Build history of the part. All positions in model axes, mm. A direction names the side the tool comes from. Give positions to 0.01 mm unless a question says otherwise; leave off trailing zeros. Order: outer loops, then holes, each group sorted by start corner. A loop starts at its lowest first (then second) coordinate and runs counter-clockwise, first axis right, second up. Notation, with made-up numbers: M 73,-34.5 L 108,-34.5 A24 cw 108,-1.5 Z; hole C -33,-38 d11. An arc over 180 degrees is marked long. One line per item, written item: value. Start each with the question number.
from build123d import *

# Parameters (mm, degrees)
F1_DEPTH = 2.6162
F2_W     = 9.779
F2_H     = 9.779
F3_DEPTH = 25
F4_R     = 0.762


with BuildPart() as f1:
    # F0 (on Front) → F1 (new body)
    with BuildSketch(Plane.XZ):
        with BuildLine():
            ThreePointArc((20.4, 0), (21.66188, 12.943724), (25.4, 25.4))
            ThreePointArc((25.4, 25.4), (12.943724, 21.66188), (0, 20.4))
            ThreePointArc((0, 20.4), (-12.943724, 21.66188), (-25.4, 25.4))
            ThreePointArc((-25.4, 25.4), (-20.4, 0), (-25.4, -25.4))
            ThreePointArc((-25.4, -25.4), (0, -20.4), (25.4, -25.4))
            ThreePointArc((25.4, -25.4), (21.66188, -12.943724), (20.4, 0))
        make_face()
    extrude(amount=F1_DEPTH)

    # F2 (on face) → F3 (cut)
    with BuildSketch(Plane(origin=(0, 0, 0), x_dir=(-1, 0, 0), z_dir=(0, 1, 0))):
        Rectangle(F2_W, F2_H)
    extrude(amount=-F3_DEPTH, mode=Mode.SUBTRACT)

    # F4
    f4_edges = [f1.edges().sort_by_distance(p)[0] for p in [
        (25.4, -1.3081, 25.4),
        (-25.4, -1.3081, 25.4),
        (-25.4, -1.3081, -25.4),
        (25.4, -1.3081, -25.4),
    ]]
    fillet(f4_edges, radius=F4_R)


solid = f1.part
1) Pull direction Z, two halves, no side cores. Call faces 1 (the flat face through (0, -1, -4.89)), 2 (the cylindrical face through (-0.3, -1.3, -20.4)), 3 (the flat face through (5.2, 0, 0.3)): pulls with the +Z half, pulls with the -Z half, needs draft (parallel to the pull), parting line crosses it, or undercut.
2) Slice it at A-A (x = -2.5). List the corners of the cut face in (y, z).
3) Slice it at C-C (x = 11.5). List the corners of the cut face in (y, z), plus the area to 3 significant figures.
4) Drill centre lines: line 1 (X direction, y = -0.2, z = 1); line 2 (X direction, y = -1.9, z = 3.5); line 3 (Z direction, x = -2, y = -1.7). Where is each one in solid material? Low to high.
5) Slice it at B-B (z = 9.5). List the corners of the cut face in (x, y), plus the area to 3 significant figures.
6) Tool access for faces 4 (the cylindrical face through (-20.4, -1.3, 0.3)), 5 (the flat face through (4.89, -1, 0)): list every direction of +Z, -Z, +X, -X, +Y, -Y with a clear straight run to the whole face (end or side of a thin tool).
7) Drop flat-ended pins along their axis: P1, Ø1.3, axis at y = -1, z = 2, coming from the -X side; P2, Ø0.8, axis at y = -1, z = -2, coming from the +X side; P3, Ø0.8, axis at x = -2.5, y = -1.5, coming from the -Z side. Give the stop position or say it passes through.
Results list:
1. face 1: undercut
1. face 2: pulls with the -Z half
1. face 3: needs draft
2. outline: M -2.62,-20.45 L 0,-20.45 L 0,-4.89 L -2.62,-4.89 Z; M -2.62,4.89 L 0,4.89 L 0,20.45 L -2.62,20.45 Z
3. outline: M -2.62,-21.39 L 0,-21.39 L 0,21.39 L -2.62,21.39 Z
3. area: 112 mm²
4. line 1: x = -20.41 to -4.89, 4.89 to 20.41
4. line 2: x = -20.49 to -4.89, 4.89 to 20.49
4. line 3: z = -20.43 to -4.89, 4.89 to 20.43
5. outline: M -21.08,-2.62 L 21.08,-2.62 L 21.08,0 L -21.08,0 Z
5. area: 110 mm²
6. face 4: -X, +Y, -Y
6. face 5: +Y, -Y
7. P1: stops at x = -20.45
7. P2: stops at x = 20.44
7. P3: stops at z = -20.46
